The listing builds one solid part. Answer for the finished solid, in the listing's coordinates (mm). A direction names the side the tool comes from. Coordinates: 2 decimals unless noted, no trailing zeros. Loops run counter-clockwise (first coordinate to the right, second up) from the corner with the lowest first, then second, coordinate; pieces in that order, holes last. Notation, with made-up numbers: M 13,-2 L 50,-2 A15 ccw 50,16 Z; hole C 41,7.25 d4. An arc over 180 degrees is marked long. Answer in a Markdown table with one row per item. Add a question column.
Autodesk Inventor part; units mm, degrees
ref_plane "YZ Plane" through (0, 0, 0) normal (1, 0, 0) x (0, 1, 0)
ref_plane "XZ Plane" through (0, 0, 0) normal (0, 1, 0) x (-1, 0, 0)
ref_plane "XY Plane" through (0, 0, 0) normal (0, 0, 1) x (1, 0, 0)
sketch "Sketch1" plane through (0, 0, 0) normal (0, 1, 0) x (-1, 0, 0)
  line L0 (173.4504, -76.1021) -> (92.9116, -76.1021)
  line L1 (92.9116, -76.1021) -> (92.9116, 0)
  line L2 (92.9116, 0) -> (173.4504, 0)
  line L3 (173.4504, 0) -> (173.4504, -76.1021)
  point P0 (0, 0)
extrude "Extrusion1" add sketch "Sketch1" along normal blind 6.35
fillet "Fillet1" radius 7.62 4 edges at (-173.4504, 3.175, 0) (-173.4504, 3.175, -76.1021) (-92.9116, 3.175, -76.1021) (-92.9116, 3.175, 0)
sketch "Sketch2" plane through (0, 6.35, 0) normal (0, 1, 0) x (1, 0, 0)
  arc A0 (-165.8304, 76.1021) -> (-173.4504, 68.4821) centre (-165.8304, 68.4821) ccw
  line L0 (-100.5316, 76.1021) -> (-165.8304, 76.1021)
  circle A1 centre (-165.8304, 68.4821) radius 7.62
  arc A2 (-173.4504, 7.62) -> (-165.8304, 0) centre (-165.8304, 7.62) ccw
  circle A3 centre (-165.8304, 7.62) radius 7.62
  arc A4 (-100.5316, 0) -> (-92.9116, 7.62) centre (-100.5316, 7.62) ccw
  circle A5 centre (-100.5316, 7.62) radius 7.62
  arc A6 (-92.9116, 68.4821) -> (-100.5316, 76.1021) centre (-100.5316, 68.4821) ccw
  circle A7 centre (-100.5316, 68.4821) radius 7.62
  line L1 (-169.6404, 72.2921) -> (-96.7216, 72.2921)
  line L2 (-96.7216, 72.2921) -> (-96.7216, 3.81)
  line L3 (-96.7216, 3.81) -> (-169.6404, 3.81)
  line L4 (-169.6404, 3.81) -> (-169.6404, 72.2921)
  line L5 (-173.4504, 68.4821) -> (-173.4504, 7.62)
  point P0 (0, 0)
  point P1 (-169.6404, 38.051)
  point P2 (-173.4504, 38.051)
  point P3 (-133.181, 72.2921)
  point P4 (-133.181, 76.1021)
  point P5 (-169.6404, 61.8829)
  point P6 (-169.6404, 14.2191)
  point P7 (-159.2312, 3.81)
  point P8 (-107.1307, 3.81)
  point P9 (-96.7216, 14.2191)
  point P10 (-96.7216, 61.8829)
  point P11 (-107.1307, 72.2921)
  point P12 (-159.2312, 72.2921)
  dimension "d3" = 3.81
  dimension "d4" = 3.81
extrude "Extrusion2" cut sketch "Sketch2" against normal blind 2.54 contours L1 A7 L2 A5 L3 A3 L4 A1
fillet "Fillet2" radius 7.62 8 edges at (-169.6404, 5.08, -14.2191) (-159.2312, 5.08, -3.81) (-169.6404, 5.08, -61.8829) (-159.2312, 5.08, -72.2921) (-107.1307, 5.08, -72.2921) (-96.7216, 5.08, -61.8829) (-96.7216, 5.08, -14.2191) (-107.1307, 5.08, -3.81)
fillet "Fillet3" radius 2.54 16 edges at (-155.7406, 3.81, -5.4059) (-160.4422, 3.81, -13.0082) (-168.0445, 3.81, -17.7098) (-169.6404, 3.81, -38.051) (-168.0445, 3.81, -58.3923) (-160.4422, 3.81, -63.0939) (-155.7406, 3.81, -70.6962) (-133.181, 3.81, -72.2921) (-110.6214, 3.81, -70.6962) (-105.9198, 3.81, -63.0939) (-98.3175, 3.81, -58.3923) (-96.7216, 3.81, -38.051) (-98.3175, 3.81, -17.7098) (-105.9198, 3.81, -13.0082) (-110.6214, 3.81, -5.4059) (-133.181, 3.81, -3.81)
equation "\"d4\" = d3"
properties part number "Machined Lid" material "Aluminum 6061"
(1) For faces 1 (the face through (-95.085, 3.219, -73.811)), 2 (the face through (-168.916, 4.574, -37.832)), determine the directions among +Z, -Z, +X, -X, +Y, -Y from which every point of the face is accessible in a straight line to the end or side of a thin tool.
(2) This flat-tipped pin is pushed along its axis until it touches: pin 1 (5 mm diameter, centred on x = -127, z = -39.5, fed in from +Y). Where does it stop, or does it pass through?
(3) A cutting plane is placed at C-C (y = 4.75). Give the vertices of the cut face in (x, z), plus the area to 3 significant figures.
(4) The mould has two halves that part along X. Classify faces 3 (the face through (-133, 0, -38)), 4 (the face through (-173.45, 3, -38)), 5 (the face through (-97.45, 4.57, -38.27)): released by +X, released by -X, zero draft, split by the parting line, or undercut.
(5) Straight lines are drawn through the part: line 1 (Y direction, x = -153, z = -24); line 2 (X direction, y = 5, z = -7.5); line 3 (X direction, y = 5.75, z = -52). For each, find the intervals that lie inside material, in ascending order.
Solved:
| question | item | result |
|---|---|---|
| 1 | face 1 | -Z, +X, +Y, -Y |
| 1 | face 2 | +Y |
| 2 | pin 1 | stops at y = 3.81 |
| 3 | outline | M -173.45,-68.48 A7.62 ccw -165.83,-76.1 L -100.53,-76.1 A7.62 ccw -92.91,-68.48 L -92.91,-7.62 A7.62 ccw -100.53,0 L -165.83,0 A7.62 ccw -173.45,-7.62 Z; hole M -169.07,-53.73 A7.05 ccw -163.78,-60.56 A8.19 cw -157.9,-66.44 A7.05 ccw -151.07,-71.73 L -115.29,-71.73 A7.05 ccw -108.46,-66.44 A8.19 cw -102.58,-60.56 A7.05 ccw -97.29,-53.73 L -97.29,-22.38 A7.05 ccw -102.58,-15.55 A8.19 cw -108.46,-9.67 A7.05 ccw -115.29,-4.38 L -151.07,-4.38 A7.05 ccw -157.9,-9.67 A8.19 cw -163.78,-15.55 A7.05 ccw -169.07,-22.38 Z |
| 3 | area | 1,780 mm² |
| 4 | face 3 | zero draft |
| 4 | face 4 | released by -X |
| 4 | face 5 | undercut |
| 5 | line 1 | y = 0 to 3.81 |
| 5 | line 2 | x = -173.45 to -157.15, -109.22 to -92.91 |
| 5 | line 3 | x = -173.45 to -169.57, -96.79 to -92.91 |
